Autodesk Inventor part; units mm, degrees
ref_plane "XY Plane" through (0, 0, 0) normal (0, 0, 1) x (1, 0, 0)
sketch "Block1" plane through (0, 0, 0) normal (0, 0, 1) x (1, 0, 0)
  line L0 (-0.685, 86) -> (2.315, 86)
  line L1 (-0.685, 86) -> (-0.685, 91)
  line L2 (2.315, 86) -> (1.4022, 87.742)
  line L3 (1.4022, 87.742) -> (1.4022, 89)
  line L4 (-0.5978, 91) -> (-0.685, 91)
  arc A0 (1.4022, 89) -> (-0.5978, 91) centre (-0.5978, 89) ccw
  point P0 (0.6511, 88.4856)
  dimension "d9" = 3
  dimension "d10" = 5
  dimension "d11" = 2
  dimension "d14" = 152.344
  dimension "d15" = 2.0871
sketch "Skizze1" plane through (0, 0, 0) normal (0, 0, 1) x (1, 0, 0)
  point P0 (0, 0)
sketch "Skizze2" plane through (0, 0, 0) normal (0, 0, 1) x (1, 0, 0)
  circle A0 centre (0, 0) radius 11.25
  dimension "d0" = 22.5
extrude "Extrusion1" add sketch "Skizze2" along normal blind 30
sketch "Skizze3" plane through (0, 0, 30) normal (0, 0, 1) x (1, 0, 0)
  circle A0 centre (0, 0) radius 11.25
  circle A1 centre (0, 0) radius 5
  dimension "d3" = 10
extrude "Extrusion2" add sketch "Skizze3" along normal blind 7 contours A1
sketch "Skizze4" plane through (0, 0, 37) normal (0, 0, 1) x (1, 0, 0)
  circle A0 centre (0, 0) radius 5
  circle A1 centre (0, 0) radius 2.5
  dimension "d6" = 5
extrude "Extrusion3" add sketch "Skizze4" along normal blind 6 contours A1
sketch "Skizze5" plane through (0, 0, 0) normal (1, 0, 0) x (0, 1, 0)
  line L0 (2.5, 43) -> (-2.5, 43)
  line L1 (-2.5, 43) -> (2.5, 43) construction
  line L2 (0, 43) -> (3, 43)
  line L3 (0, 43) -> (0, 48)
  line L4 (3, 43) -> (2.0871, 44.742)
  line L5 (2.0871, 44.742) -> (2.0871, 46)
  line L6 (0.0871, 48) -> (0, 48)
  arc A0 (2.0871, 46) -> (0.0871, 48) centre (0.0871, 46) ccw
  point P0 (0, 0)
sketch "Skizze6" plane through (0, 0, 0) normal (0, 0, -1) x (-1, 0, 0)
  line L0 (7, 3.5) -> (7, -3.5)
  line L1 (7, -3.5) -> (8, -3.5)
  line L2 (7, 3.5) -> (8, 3.5)
  line L3 (8, -3.5) -> (8, 3.5)
  line L4 (0, 11.25) -> (0, -11.25) construction
  line L5 (-7, 3.5) -> (-7, -3.5)
  line L6 (-7, -3.5) -> (-8, -3.5)
  line L7 (-7, 3.5) -> (-8, 3.5)
  line L8 (-8, -3.5) -> (-8, 3.5)
  point P0 (0, 0)
  dimension "d19" = 7
  dimension "d20" = 1
  dimension "d21" = 7
  dimension "d23" = 3.5
extrude "Extrusion4" add sketch "Skizze6" along normal blind 10
revolve "Umdrehung2" add sketch "Skizze5" angle 360 about axis through (0, 0, 43) along (0, 0, 1)
ref_plane "Arbeitsebene2" through (0, 5, 30) normal (0, 1, 0) x (-1, 0, 0)
ref_plane "Arbeitsebene1" through (0, 5, 30) normal (0, 1, 0) x (-1, 0, 0)
sketch "Skizze7" plane through (0, 5, 30) normal (0, 1, 0) x (-1, 0, 0)
  circle A0 centre (0, 3.4888) radius 2.5
  point P0 (0, -30)
  dimension "d27" = 5
extrude "Extrusion5" add sketch "Skizze7" along normal blind 15 and the other way blind 3
sketch "Skizze9" plane through (0, 0, 0) normal (1, 0, 0) x (0, 1, 0)
  point P0 (0, 0)
sketch "Skizze10" plane through (0, 0, 0) normal (1, 0, 0) x (0, 1, 0)
  point P0 (0, 0)
ref_plane "Arbeitsebene6" through (0, 0, 0) normal (1, 0, 0) x (0, 1, 0)
ref_plane "Arbeitsebene7" through (0, 20, 33.4888) normal (0, 1, 0) x (1, 0, 0)
sketch "Skizze11" plane through (0, 0, 0) normal (1, 0, 0) x (0, 1, 0)
  point P0 (0, 0)
sketch "Skizze12" plane through (0, 0, 0) normal (1, 0, 0) x (0, 1, 0)
  line L0 (0, 0) -> (0, 41.8024) construction
sketch "Skizze13" plane through (0, 0, 0) normal (1, 0, 0) x (0, 1, 0)
  line L0 (0, 43) -> (3, 43)
  line L1 (0, 43) -> (0, 48)
  line L2 (3, 43) -> (2.0871, 44.742)
  line L3 (2.0871, 44.742) -> (2.0871, 46)
  line L4 (0.0871, 48) -> (0, 48)
  arc A0 (2.0871, 46) -> (0.0871, 48) centre (0.0871, 46) ccw
  line L5 (19.9907, 33.5038) -> (19.9907, 30.5038)
  line L6 (19.9907, 33.5038) -> (24.9907, 33.5038)
  line L7 (19.9907, 30.5038) -> (21.7326, 31.4166)
  line L8 (21.7326, 31.4166) -> (22.9907, 31.4166)
  line L9 (24.9907, 33.4166) -> (24.9907, 33.5038)
  arc A1 (22.9907, 31.4166) -> (24.9907, 33.4166) centre (22.9907, 33.4166) ccw
  point P0 (0, 0)
revolve "Umdrehung3" add sketch "Skizze13" angle 360 about axis through (0, 19.9907, 33.5038) along (0, 1, 0) contours L6 L9 A1 L8 L7 L5
fillet "Rundung1" radius 2 1 edges at (-11.25, 0, 30)
ref_plane "Arbeitsebene8" through (0, 0.0871, 48) normal (0, 0, 1) x (1, 0, 0)
sketch "Skizze14" plane through (0, 0.0871, 48) normal (0, 0, 1) x (1, 0, 0)
  point P0 (0, -0.0871)
  point P1 (0, -0.0871)
hole "Bohrung1" at (0, 0, 48) direction (0, 0, -1) diameter 3 depth 15 tip angle 118
ref_plane "Arbeitsebene9" through (0, 24.9907, 33.4166) normal (0, 1, 0) x (-1, 0, 0)
sketch "Skizze15" plane through (0, 24.9907, 33.4166) normal (0, 1, 0) x (-1, 0, 0)
  point P0 (0, -33.4166)
  point P1 (0, 0)
hole "Bohrung2" at (0, 24.9907, 33.4166) direction (0, -1, 0) diameter 3 depth 20 tip angle 118
properties part number "Ventil"
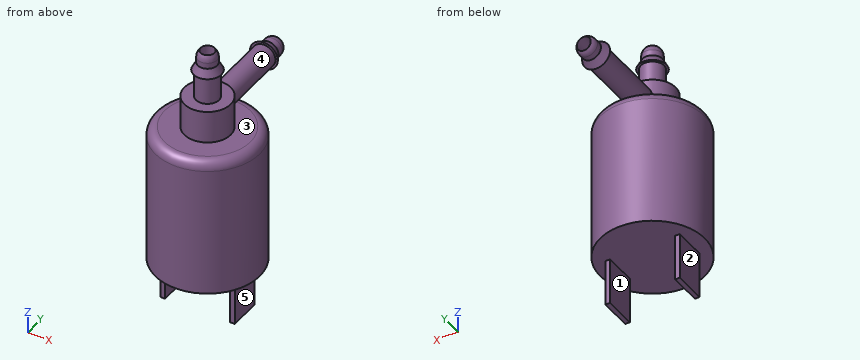
The model under review builds one solid part; all positions refer to its coordinate system, in mm. Face numbers are marked on the shaded views. A direction names the side the tool comes from. Round coordinates to 2 decimals unless told otherwise and drop trailing zeros. Loops run counter-clockwise (first coordinate to the right, second up) from the corner with the lowest first, then second, coordinate; pieces in that order, holes last. Notation, with made-up numbers: (44, 86.5) -> (81, 86.5) arc R23 ccw to (81, 108.5) -> close; hole circle Ø5 at (21.25, 50). An arc over 180 degrees is marked (long way). Write item = value, one per line. Start each with the question number.
Item 1: For the marked faces 1, 2 and 3, list the 3-axis set-ups (+Z, -Z, +X, -X, +Y, -Y) from which the entire face can be reached by the end or side of a thin tool; tool diameter is ignored.
Item 2: Mouldability with a two-part tool opening along Z and no side actions: class the marked faces 4 and 5 as released by +Z, released by -Z, zero draft, split by the parting line, or undercut.
Item 3: Insertion check: pin 1 (2 mm diameter, centred on y = 0.5, z = -5, fed in from +X); pin 2 (2.5 mm diameter, centred on x = 0, y = 0, fed in from +Z); pin 3 (6 mm diameter, centred on y = 10, z = 16, fed in from -X); pin 4 (2 mm diameter, centred on x = 7.5, z = 37, fed in from -Y). Each pin has a flat end and moves straight along its axis. Give the tip position at first contact, or say it passes through.
Item 4: Take a section at A-A on z = 3. Give the boundary of the cut face in (x, y).
Item 5: Take a section at B-B on y = 18.5. Give the boundary of the cut face in (x, z), plus the area to 3 significant figures.
Item 6: To check wall thickness, follow L1, parallel to Y at x = 0, z = 38.25; L2, parallel to Z at x = 0, y = 15.25; L3, parallel to Z at x = 1, y = 5. State the ranges of each line that lie inside material, in increasing order.
Result:
q1.face_1 = -Z, +Y, -Y
q1.face_2 = -Z, -X, +Y, -Y
q1.face_3 = none
q2.face_4 = undercut
q2.face_5 = zero draft
q3.pin_1 = 8
q3.pin_2 = 32.85
q3.pin_3 = -8.81
q3.pin_4 = through
q4.outline = circle Ø22.5 at (0, 0)
q5.outline = circle Ø5 at (0, 33.49); hole circle Ø3 at (0, 33.42)
q5.area = 12.6 mm²
q6.L1 = -2.5 to -1.5, 1.5 to 2.5
q6.L2 = 30.99 to 31.92, 34.92 to 35.99
q6.L3 = 0 to 30, 31.2 to 32.3, 34.53 to 35.78
